```python
from build123d import *

# Parameters (mm, degrees)
SKETCH_R      = 4.5
SKETCH_R_2    = 2.8
PAD_DEPTH     = 2
SKETCH001_R   = 10
SKETCH001_R_2 = 1.65
PAD001_DEPTH  = 2.5
SKETCH002_R   = 1.65
POCKET_DEPTH  = 4.501


with BuildPart() as part:
    # Sketch → Pad (new body)
    with BuildSketch(Plane.XY):
        Circle(SKETCH_R)
        Circle(SKETCH_R_2, mode=Mode.SUBTRACT)
    extrude(amount=PAD_DEPTH)

    # Sketch001 (on Face4 of Pad) → Pad001 (join)
    with BuildSketch(Plane.XY.offset(2)):
        Circle(SKETCH001_R)
        Circle(SKETCH001_R_2, mode=Mode.SUBTRACT)
    extrude(amount=PAD001_DEPTH)

    # Sketch002 (on Face7 of Pad001) → Pocket (cut, through all)
    with BuildSketch(Plane.XY.offset(4.5)):
        with Locations((-7.3, 0)):
            Circle(SKETCH002_R)
        with Locations((0, -7.3)):
            Circle(SKETCH002_R)
        with Locations((0, 7.3)):
            Circle(SKETCH002_R)
        with Locations((7.3, 0)):
            Circle(SKETCH002_R)
    extrude(amount=-POCKET_DEPTH, mode=Mode.SUBTRACT)


solid = part.part
```
Part model, mm, in its own coordinate system. A direction names the side the tool comes from. Round coordinates to 2 decimals unless told otherwise and drop trailing zeros. Order: outer loops, then holes, each group sorted by start corner. A loop starts at its lowest first (then second) coordinate and runs counter-clockwise, first axis right, second up. Notation, with made-up numbers: M 31.25,-8.5 L 72.25,-8.5 A17 ccw 72.25,-3.5 Z; hole C 89,7 d3. An arc over 180 degrees is marked long. Answer in a Markdown table with one row per item. Add a question column.
Q1. Pin check, flat tips, straight feed: pin 1 (3 mm diameter, centred on x = 0, y = 7.3, fed in from -Z); pin 2 (5.5 mm diameter, centred on x = 7.3, y = 0, fed in from -Z); pin 3 (1.5 mm diameter, centred on y = -7.5, z = 3.5, fed in from +X). Stop position of each tip, or through.
Q2. 3-axis set-ups, long thin cutter, end or side, ignore diameter. For faces 4 (the face through (0, 5, 2)), 5 (the face through (0, -2, 4.5)): which of +Z, -Z, +X, -X, +Y, -Y reach the whole face in a straight line?
Q3. Wall check: L1, parallel to Y at x = 0, z = 3.45; L2, parallel to Y at x = 0, z = 1.2; L3, parallel to Z at x = 5.5, y = 4. Give the ranges that are in metal, low to high. Write a range as from..to.
Q4. Cut at D-D on y = 7.3. Give the cut face in (x, z).
Q5. Cut at A-A on y = 0. Give the cut face in (x, z).
Q6. Cut at C-C on z = 3.95. Give the cut face in (x, y), and give its area (3 significant figures).
Q7. Mould opens along Y. For faces 1 (the face through (0, -3, 0)), 2 (the face through (-2.17, -9.76, 3.23)), 3 (the face through (-2.8, 0.1, 1)) say: +Y half, -Y half, draft (parallel to the pull), parting line (faces both ways), or undercut.
Established:
| question | item | result |
|---|---|---|
| 1 | pin 1 | passes through |
| 1 | pin 2 | stops at z = 2 |
| 1 | pin 3 | stops at x = 7.38 |
| 2 | face 4 | -Z |
| 2 | face 5 | +Z, +X, -X, +Y, -Y |
| 3 | L1 | y = -10..-8.95, -5.65..-1.65, 1.65..5.65, 8.95..10 |
| 3 | L2 | y = -4.5..-2.8, 2.8..4.5 |
| 3 | L3 | z = 2..4.5 |
| 4 | outline | M -6.83,2 L -1.65,2 L -1.65,4.5 L -6.83,4.5 Z; M 1.65,2 L 6.83,2 L 6.83,4.5 L 1.65,4.5 Z |
| 5 | outline | M -10,2 L -8.95,2 L -8.95,4.5 L -10,4.5 Z; M -5.65,2 L -4.5,2 L -4.5,0 L -2.8,0 L -2.8,2 L -1.65,2 L -1.65,4.5 L -5.65,4.5 Z; M 1.65,2 L 2.8,2 L 2.8,0 L 4.5,0 L 4.5,2 L 5.65,2 L 5.65,4.5 L 1.65,4.5 Z; M 8.95,2 L 10,2 L 10,4.5 L 8.95,4.5 Z |
| 6 | outline | C 0,0 d20; hole C -7.3,0 d3.3; hole C 0,-7.3 d3.3; hole C 0,0 d3.3; hole C 0,7.3 d3.3; hole C 7.3,0 d3.3 |
| 6 | area | 271 mm2 |
| 7 | face 1 | draft |
| 7 | face 2 | parting line |
| 7 | face 3 | undercut |
